Could you check a few things on this model? Use its own coordinates, in mm. Face numbers are marked on the shaded views. A direction names the side the tool comes from. Round coordinates to 2 decimals unless told otherwise and drop trailing zeros. Loops run counter-clockwise (first coordinate to the right, second up) from the corner with the lowest first, then second, coordinate; pieces in that order, holes last. Notation, with made-up numbers: M 34,39.5 L 65,39.5 A13 ccw 65,63.5 Z; hole C 81,-21.75 d8. An arc over 180 degrees is marked long. Return JSON: item names as keys, results as strings. Group by question number.
```python
from build123d import *


with BuildPart() as f1:
    # F0 (on Front) → F1 (revolve)
    with BuildSketch(Plane.XZ):
        Polygon((22.86, 39.777045), (22.86, 50.445045), (0, 50.445045), (0, -51.154955), (22.86, -51.154955), (22.86, -40.486955), (10.16, -18.288), (10.16, -7.62), align=None)
    revolve(axis=Axis((0, 0, -0.354955), (0, 0, 1)))

    # F2 (on Front) → F3 (revolve, cut)
    with BuildSketch(Plane.XZ):
        with BuildLine():
            Line((10.439722, -2.650541), (21.844, 39.910804))
            Line((21.844, 39.910804), (21.844, 50.445045))
            Line((21.844, 50.445045), (0, 50.445045))
            Line((0, 50.445045), (0, -7.35704))
            Line((0, -7.35704), (4.306093, -7.35704))
            ThreePointArc((4.306093, -7.35704), (8.171728, -6.044834), (10.439722, -2.650541))
        make_face()
    revolve(axis=Axis((0, 0, 21.544003), (0, 0, 1)), mode=Mode.SUBTRACT)

    # F4 (on Front) → F5 (revolve, cut)
    with BuildSketch(Plane.XZ):
        with BuildLine():
            Line((21.844, -40.757043), (11.134297, -22.037026))
            ThreePointArc((11.134297, -22.037026), (8.808393, -19.697309), (5.622545, -18.840293))
            Line((5.622545, -18.840293), (0, -18.840293))
            Line((0, -18.840293), (0, -51.154955))
            Line((0, -51.154955), (21.844, -51.154955))
            Line((21.844, -51.154955), (21.844, -40.757043))
        make_face()
    revolve(axis=Axis((0, 0, -34.997624), (0, 0, -1)), mode=Mode.SUBTRACT)


solid = f1.part
```
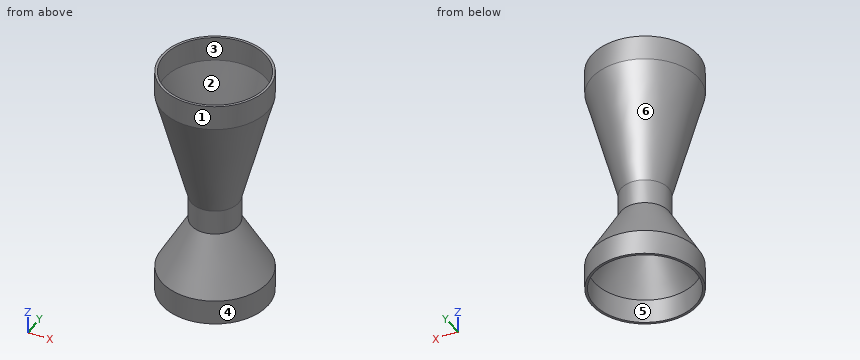
1. We'd pull the mould along X, two halves only. Please class the marked faces 1 and 2: +X half, -X half, draft (parallel to the pull), parting line (faces both ways), or undercut.
2. If we section it at A-A, the plane z = 14: Please give me the cut outline in (x, y), then the cut area to 3 significant figures.
3. I'm going to push flat-ended pins straight in: pin 1 Ø4 at (x, y) = (8, 1.5) entering from +Z; pin 2 Ø5 at (x, y) = (-4.5, -18) entering from -Z; pin 3 Ø12 at (x, y) = (13.5, -5) entering from -Z. Where does each tip first touch, or does it pass through?
4. I need wall thicknesses on probe 1 along Y at (x, z) = (0, 43); probe 2 along X at (y, z) = (18.5, -40.5); probe 3 along Y at (x, z) = (-5, 8). Which ranges of each line are inside material? Lowest first, please.
5. On a 3-axis mill with a long thin cutter (end or side, diameter ignored), from which of +Z, -Z, +X, -X, +Y, -Y can I reach the whole of each face in a straight line? I mean the marked faces 3, 4, 5 and 6. Say none if no direction works.
Geometry results:
{
 "1": {"face 1": "parting line", "face 2": "undercut"},
 "2": {"outline": "C 0,0 d31.91; hole C 0,0 d29.8", "area": "102 mm^2"},
 "3": {"pin 1": "z = -3.52", "pin 2": "z = -39.38", "pin 3": "z = -38.23"},
 "4": {"probe 1": "-22.86 to -21.84, 21.84 to 22.86", "probe 2": "-13.43 to -11.34, 11.34 to 13.43", "probe 3": "-13.45 to -12.32, 12.32 to 13.45"},
 "5": {"face 3": "+Z", "face 4": "+Z, -Z", "face 5": "-Z", "face 6": "none"}
}
